The listing builds one solid part. Answer for the finished solid, in the listing's coordinates (mm). Face numbers are marked on the shaded views. Give positions to 0.01 mm unless a question says otherwise; leave off trailing zeros. Write each loop counter-clockwise with the first axis right and the second up, starting at its lowest first coordinate (ties: lowest second). Pieces come first, ordered by that corner, then holes.
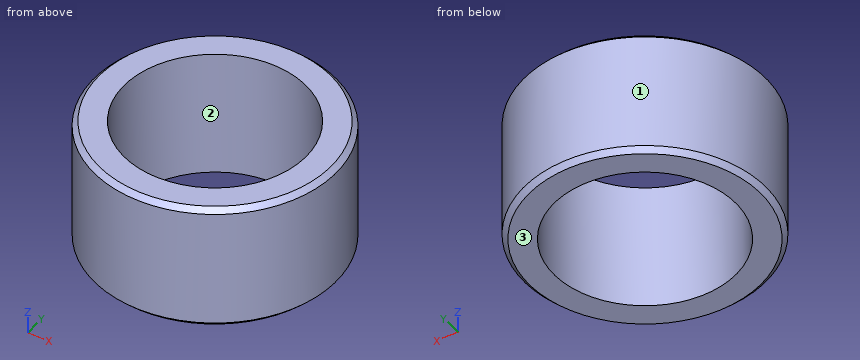
Autodesk Inventor part; units mm, degrees
ref_plane "YZ Plane" through (0, 0, 0) normal (1, 0, 0) x (0, 1, 0)
ref_plane "XZ Plane" through (0, 0, 0) normal (0, 1, 0) x (-1, 0, 0)
ref_plane "XY Plane" through (0, 0, 0) normal (0, 0, 1) x (1, 0, 0)
sketch "Sketch1" plane through (0, 0, 0) normal (0, 0, 1) x (1, 0, 0)
  circle A0 centre (0, 0) radius 4.85
  dimension "d0" = 9.7
extrude "Extrusion1" add sketch "Sketch1" against normal blind 5.1
sketch "Sketch2" plane through (0, 0, 0) normal (0, 0, 1) x (1, 0, 0)
  circle A0 centre (0, 0) radius 3.65
  dimension "d3" = 7.3
extrude "Extrusion2" cut sketch "Sketch2" against normal through all
chamfer "Chamfer1" distance 0.2 angle 45 2 edges at (-4.85, 0, 0) (-4.85, 0, -5.1)
properties part number "cap_bot"
Item 1: A cutting plane is placed at C-C, the plane z = -3.6. Give the vertices of the cut face in (x, y).
Conclusion:
outline: circle Ø9.7 at (0, 0); hole circle Ø7.3 at (0, 0)
Item 2: A cutting plane is placed at A-A, the plane y = 0. Give the vertices of the cut face in (x, z).
Conclusion:
outline: (-4.85, -4.9) - (-4.65, -5.1) - (-3.65, -5.1) - (-3.65, 0) - (-4.65, 0) - (-4.85, -0.2) - close; (3.65, -5.1) - (4.65, -5.1) - (4.85, -4.9) - (4.85, -0.2) - (4.65, 0) - (3.65, 0) - close
Item 3: Consider probe 1 along Y at (x, z) = (0, -0.55); probe 2 along Y at (x, z) = (1.25, -3.35); probe 3 along X at (y, z) = (0.5, -2.2). Determine where each line is inside the solid, lowest interval first.
Conclusion:
probe 1: y = -4.85 to -3.65, 3.65 to 4.85
probe 2: y = -4.69 to -3.43, 3.43 to 4.69
probe 3: x = -4.82 to -3.62, 3.62 to 4.82
Item 4: Determine the mould class of the marked faces 1, 2 and 3 for opening direction X: pulls with the +X half, pulls with the -X half, needs draft (parallel to the pull), parting line crosses it, or undercut.
Conclusion:
face 1: parting line crosses it
face 2: undercut
face 3: needs draft
Item 5: This flat-tipped pin is pushed along its axis until it touches: P1, Ø2, axis at x = 1.5, z = -1, coming from the +Y side. Where does it stop, or does it pass through?
Conclusion:
P1: stops at y = 4.82
